from build123d import *

# Parameters (mm, degrees)
SKETCH_W   = 45
SKETCH_H   = 8
SKETCH_W_2 = 18
SKETCH_H_2 = 2
PAD_DEPTH  = 15


with BuildPart() as part:
    # Sketch → Pad (new body)
    with BuildSketch(Plane.XZ):
        with Locations((22.5, 4)):
            Rectangle(SKETCH_W, SKETCH_H)
        with Locations((12, 4)):
            Rectangle(SKETCH_W_2, SKETCH_H_2, mode=Mode.SUBTRACT)
        with Locations((33, 4)):
            Rectangle(SKETCH_W_2, SKETCH_H_2, mode=Mode.SUBTRACT)
    extrude(amount=PAD_DEPTH)


solid = part.part
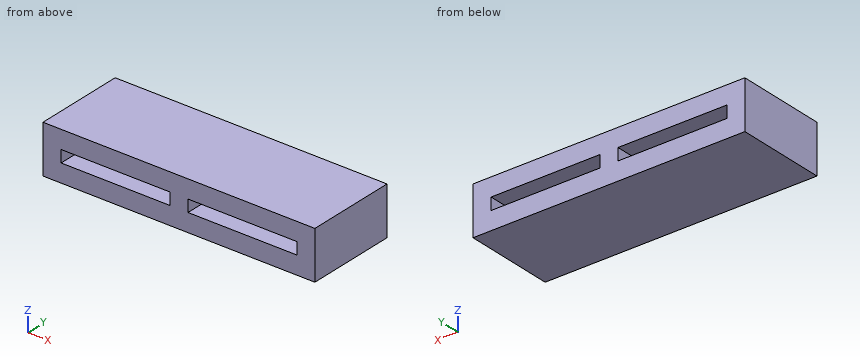
Here's how the part is built. I have some questions about the finished solid (model axes, mm). Give positions to 0.01 mm unless a question says otherwise; leave off trailing zeros. Write each loop counter-clockwise with the first axis right and the second up, starting at its lowest first coordinate (ties: lowest second). Pieces come first, ordered by that corner, then holes. Notation, with made-up numbers: (73.5, 3) -> (123.5, 3) arc R23 cw to (123.5, 37) -> close; hole circle Ø6 at (-21.75, 33.25). An arc over 180 degrees is marked (long way). Use one line per item in the form item = value. Start each with the question number.
1. If I drill on L1, parallel to X at y = -2.5, z = 3.5; L2, parallel to Z at x = 29.5, y = -3.25, over which ranges is the centre line in solid material (lowest first)?
2. Imagine slicing it at B-B on z = 4. List the corners of the cut face in (x, y) for me, plus the area to 3 significant figures.
3. Imagine slicing it at C-C on y = -3.5. List the corners of the cut face in (x, z) for me, plus the area to 3 significant figures.
4. Will this pin go through, and if not, where does the flat tip stop? pin 1 Ø0.6 at (y, z) = (-11, 4.5) entering from -X.
5. Imagine slicing it at A-A on x = 35. List the corners of the cut face in (y, z) for me.
Entries:
q1.L1 = 0 to 3, 21 to 24, 42 to 45
q1.L2 = 0 to 3, 5 to 8
q2.outline = (0, -15) -> (3, -15) -> (3, 0) -> (0, 0) -> close; (21, -15) -> (24, -15) -> (24, 0) -> (21, 0) -> close; (42, -15) -> (45, -15) -> (45, 0) -> (42, 0) -> close
q2.area = 135 mm²
q3.outline = (0, 0) -> (45, 0) -> (45, 8) -> (0, 8) -> close; hole (3, 3) -> (21, 3) -> (21, 5) -> (3, 5) -> close; hole (24, 3) -> (42, 3) -> (42, 5) -> (24, 5) -> close
q3.area = 288 mm²
q4.pin_1 = 0
q5.outline = (-15, 0) -> (0, 0) -> (0, 3) -> (-15, 3) -> close; (-15, 5) -> (0, 5) -> (0, 8) -> (-15, 8) -> close
